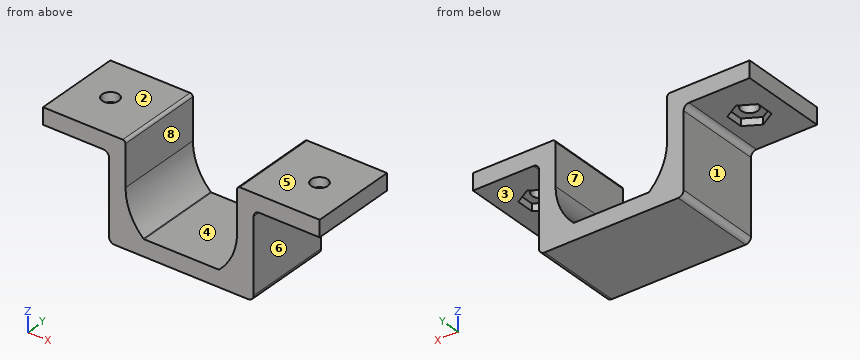
```python
from build123d import *

# Parameters (mm, degrees)
F1_DEPTH = 16
F2_R     = 1.5
F3_DEPTH = 18.501
F5_DEPTH = 1.3
F6_R     = 0.5


with BuildPart() as f1:
    # F0 (on Front) → F1 (new body)
    with BuildSketch(Plane.XZ):
        with BuildLine():
            ThreePointArc((-13.15, 1), (-12.857107, 0.292893), (-12.15, 0))
            Line((-12.15, 0), (12.15, 0))
            ThreePointArc((12.15, 0), (12.857107, 0.292893), (13.15, 1))
            Line((13.15, 1), (13.15, 14.5))
            ThreePointArc((13.15, 14.5), (13.442893, 15.207107), (14.15, 15.5))
            Line((14.15, 15.5), (25.15, 15.5))
            Line((25.15, 15.5), (25.15, 18.5))
            Line((25.15, 18.5), (13.15, 18.5))
            Line((13.15, 18.5), (10.15, 18.5))
            Line((10.15, 18.5), (10.15, 10.5))
            ThreePointArc((10.15, 10.5), (9.301266, 6.436878), (6.897004, 3.053266))
            ThreePointArc((6.897004, 3.053266), (6.834086, 3.013792), (6.761102, 3))
            Line((6.761102, 3), (-6.761102, 3))
            ThreePointArc((-6.761102, 3), (-6.834086, 3.013792), (-6.897004, 3.053266))
            ThreePointArc((-6.897004, 3.053266), (-9.301266, 6.436878), (-10.15, 10.5))
            Line((-10.15, 10.5), (-10.15, 18.5))
            Line((-10.15, 18.5), (-13.15, 18.5))
            Line((-13.15, 18.5), (-25.15, 18.5))
            Line((-25.15, 18.5), (-25.15, 15.5))
            Line((-25.15, 15.5), (-14.15, 15.5))
            ThreePointArc((-14.15, 15.5), (-13.442893, 15.207107), (-13.15, 14.5))
            Line((-13.15, 14.5), (-13.15, 1))
        make_face()
    extrude(amount=F1_DEPTH)

    # F2 (on face) → F3 (cut, through all)
    with BuildSketch(Plane.XY.offset(18.5)):
        with Locations((-19, -8)):
            Circle(F2_R)
        with Locations((19, -8)):
            Circle(F2_R)
    extrude(amount=-F3_DEPTH, mode=Mode.SUBTRACT)

    # F4 (on face) → F5 (cut)
    with BuildSketch(Plane(origin=(0, 0, 15.5), x_dir=(1, 0, 0), z_dir=(0, 0, -1))):
        Polygon((-16.2, 6.383419), (-16.2, 9.616581), (-19, 11.233162), (-21.8, 9.616581), (-21.8, 6.383419), (-19, 4.766838), align=None)
        Polygon((19, 11.233162), (16.2, 9.616581), (16.2, 6.383419), (19, 4.766838), (21.8, 6.383419), (21.8, 9.616581), align=None)
    extrude(amount=-F5_DEPTH, mode=Mode.SUBTRACT)

    # F6
    f6_edges = [f1.edges().sort_by_distance(p)[0] for p in [
        (-10.15, -8, 18.5),
        (10.15, -8, 18.5),
    ]]
    fillet(f6_edges, radius=F6_R)


solid = f1.part
```
Source: CAD feature listing. Evaluate the final solid. Frame: model axes, mm. Face numbers are marked on the shaded views. A direction names the side the tool comes from. Give positions to 0.01 mm unless a question says otherwise; leave off trailing zeros. Loops run counter-clockwise (first coordinate to the right, second up) from the corner with the lowest first, then second, coordinate; pieces in that order, holes last. Notation, with made-up numbers: (27, -19.75) - (74, -19.75) arc R22 ccw to (74, 11.25) - close; hole circle Ø2 at (37, -9). An arc over 180 degrees is marked (long way). Use CSV: the item, a comma, the result in double quotes.
1) Cut plane C-C (y = -4). Output: boundary loops of the cut face in (x, z), and give its area (3 significant figures).
Worked out:
outline,"(-25.15, 15.5) - (-14.15, 15.5) arc R1 cw to (-13.15, 14.5) - (-13.15, 1) arc R1 ccw to (-12.15, 0) - (12.15, 0) arc R1 ccw to (13.15, 1) - (13.15, 14.5) arc R1 cw to (14.15, 15.5) - (25.15, 15.5) - (25.15, 18.5) - (10.65, 18.5) arc R0.5 ccw to (10.15, 18) - (10.15, 10.5) arc R10.15 cw to (6.9, 3.05) arc R0.2 cw to (6.76, 3) - (-6.76, 3) arc R0.2 cw to (-6.9, 3.05) arc R10.15 cw to (-10.15, 10.5) - (-10.15, 18) arc R0.5 ccw to (-10.65, 18.5) - (-25.15, 18.5) - close"
area,"259 mm^2"
2) Set-up query: the marked faces 1, 2, 3 and 4. Return all of +Z, -Z, +X, -X, +Y, -Y with unobstructed straight access to the full face (end or side cutting, diameter ignored); none if empty.
Worked out:
face 1,"-Z, -X, +Y, -Y"
face 2,"+Z, +X, -X, +Y, -Y"
face 3,"-Z, +X, +Y, -Y"
face 4,"+Z, +Y, -Y"
3) Cut plane D-D (z = 6.25). Output: boundary loops of the cut face in (x, y).
Worked out:
outline,"(-13.15, -16) - (-9.22, -16) - (-9.22, 0) - (-13.15, 0) - close; (9.22, -16) - (13.15, -16) - (13.15, 0) - (9.22, 0) - close"
4) Cut plane B-B (x = 20). Output: boundary loops of the cut face in (y, z).
Worked out:
outline,"(-16, 15.5) - (-10.66, 15.5) - (-10.66, 16.8) - (-9.12, 16.8) - (-9.12, 18.5) - (-16, 18.5) - close; (-6.88, 16.8) - (-5.34, 16.8) - (-5.34, 15.5) - (0, 15.5) - (0, 18.5) - (-6.88, 18.5) - close"
5) Cut plane A-A (z = 8.75). Output: boundary loops of the cut face in (x, y).
Worked out:
outline,"(-13.15, -16) - (-10, -16) - (-10, 0) - (-13.15, 0) - close; (10, -16) - (13.15, -16) - (13.15, 0) - (10, 0) - close"
6) Line query: line 1 (X direction, y = -10.5, z = 12.5); line 2 (Y direction, x = -19, z = 17.55); line 3 (X direction, y = -12.75, z = 17.75). Output: solid intervals per line, ascending.
Worked out:
line 1,"x = -13.15 to -10.15, 10.15 to 13.15"
line 2,"y = -16 to -9.5, -6.5 to 0"
line 3,"x = -25.15 to -10.15, 10.15 to 25.15"
7) Pin query (flat end, axial travel): P1, Ø4.5, axis at x = 19, y = -9, coming from the -Z side; P2, Ø1.5, axis at y = -2, z = 3.5, coming from the +X side; P3, Ø3, axis at x = -19.5, y = -8, coming from the -Z side. Return the tip coordinate at first contact, or that it passes through.
Worked out:
P1,"stops at z = 15.5"
P2,"stops at x = 13.15"
P3,"stops at z = 16.8"
8) Mould query, pull axis X, two halves, no side actions, for the marked faces 5, 6, 7 and 8. Classes: +X half, -X half, draft (parallel to the pull), parting line (faces both ways), or undercut.
Worked out:
face 5,"draft"
face 6,"+X half"
face 7,"undercut"
face 8,"undercut"
